```python
from build123d import *

# Parameters (mm, degrees)
F1_DEPTH = 14.925
F2_R     = 2


with BuildPart() as f1:
    # F0 (on Front) → F1 (new body, symmetric)
    with BuildSketch(Plane.XZ):
        with BuildLine():
            Line((-22.5191842765, -9.075), (27.365, -9.075))
            Line((27.365, -9.075), (27.365, 9.075))
            Line((27.365, 9.075), (-22.4661100656, 9.075))
            ThreePointArc((-22.4661100656, 9.075), (-26.0623595245, 5.1465764849), (-27.3650142087, -0.0175896876))
            ThreePointArc((-27.3650142087, -0.0175896876), (-26.0774195294, -5.1537056642), (-22.5191842765, -9.075))
        make_face()
    extrude(amount=F1_DEPTH, both=True)

    # F2
    f2_edges = [f1.edges().sort_by_distance(p)[0] for p in [
        (2.449445, -14.925, 9.075),
        (2.449445, 14.925, 9.075),
        (27.365, 7.4625, 9.075),
        (27.365, -7.4625, 9.075),
        (-22.519184, 7.4625, -9.075),
        (2.422908, 14.925, -9.075),
        (27.365, 7.4625, -9.075),
        (27.365, -7.4625, -9.075),
        (2.422908, -14.925, -9.075),
        (-22.519184, -7.4625, -9.075),
        (27.365, -14.925, 0),
        (27.365, 14.925, 0),
    ]]
    fillet(f2_edges, radius=F2_R)


solid = f1.part
```
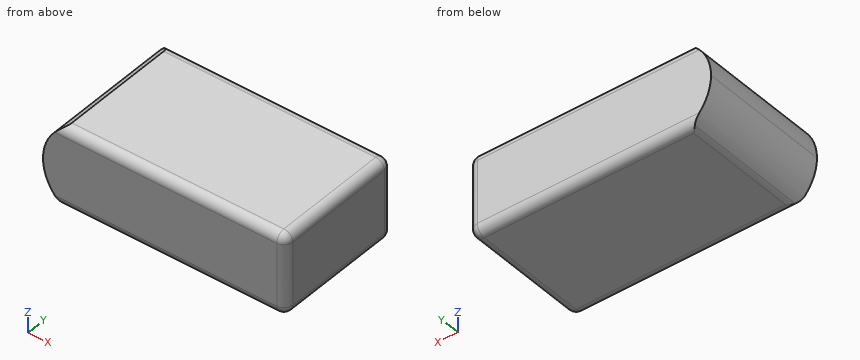
Work out the finished part from the listing and answer in its coordinate system (mm). Round coordinates to 2 decimals unless told otherwise and drop trailing zeros. Loops run counter-clockwise (first coordinate to the right, second up) from the corner with the lowest first, then second, coordinate; pieces in that order, holes last.
(1) The part is cut by section A-A, the plane y = -2.25. Give the vertices of the cut face in (x, z) (3 decimals).
Computed values:
outline: (-23.095, -8.663) arc R2 ccw to (-21.879, -9.075) - (25.365, -9.075) arc R2 ccw to (27.365, -7.075) - (27.365, 7.075) arc R2 ccw to (25.365, 9.075) - (-22.466, 9.075) arc R10.888 ccw to start
(2) The part is cut by section C-C, the plane z = -6.5. Give the vertices of the cut face in (x, y) (3 decimals), and give its area (3 significant figures).
Computed values:
outline: (-25.225, -14.925) - (25.365, -14.925) arc R2 ccw to (27.365, -12.925) - (27.365, 12.925) arc R2 ccw to (25.365, 14.925) - (-25.225, 14.925) - close
area: 1,570 mm2
(3) The part is cut by section B-B, the plane z = 6. Give the vertices of the cut face in (x, y) (3 decimals), and give its area (3 significant figures).
Computed values:
outline: (-25.551, -14.925) - (25.365, -14.925) arc R2 ccw to (27.365, -12.925) - (27.365, 12.925) arc R2 ccw to (25.365, 14.925) - (-25.551, 14.925) - close
area: 1,580 mm2
(4) Each of these flat-tipped pins is pushed along its axis until it touches: P1, Ø5, axis at y = -2, z = -3, coming from the -X side; P2, Ø1, axis at y = 8, z = 5, coming from the -X side. Where does it stop, or does it pass through?
Computed values:
P1: stops at x = -27.35
P2: stops at x = -26.38
(5) Find the intervals of material crossed by L1, parallel to Z at x = 17, y = 13; L2, parallel to X at y = 3.75, z = 0.25 (3 decimals); L3, parallel to X at y = 13.75, z = 0.75, in increasing order.
Computed values:
L1: z = -9.07 to 9.07
L2: x = -27.362 to 27.365
L3: x = -27.34 to 27.19
